```python
from build123d import *

# Parameters (mm, degrees)
SKETCH1_R           = 0.5
BOSS_EXTRUDE1_DEPTH = 2
CUT_EXTRUDE1_DEPTH  = 2
FILLET1_R           = 1
SKETCH4_W           = 2
SKETCH4_H           = 16.2
BOSS_EXTRUDE2_DEPTH = 12


with BuildPart() as part:
    # Sketch1 → Boss-Extrude1 (new body)
    # profile 1 of 3: a face of its own
    with BuildSketch(Plane(origin=(0, -1346.908376945, 0), x_dir=(1, 0, 0), z_dir=(0, 1, 0))):
        Polygon((-1025.832273514, 2000), (-1025.832273514, 1981.9), (-1023.832273514, 1981.9), (-1023.832273514, 2004), (-1027.832273514, 2004), (-1027.832273514, 2002), (-1068.432273514, 2002), (-1068.432273514, 2004), (-1072.432273514, 2004), (-1072.432273514, 1991.5), (-1070.432273514, 1991.5), (-1070.432273514, 2000), align=None)
        with Locations(Location((-1070.432273514, 2002, 0), (0, 0, 270))):
            Circle(SKETCH1_R, mode=Mode.SUBTRACT)
        with Locations(Location((-1025.832273514, 2002, 0), (0, 0, 270))):
            Circle(SKETCH1_R, mode=Mode.SUBTRACT)
    # profile 2 of 3: a face of its own
    with BuildSketch(Plane(origin=(0, -1346.908376945, 0), x_dir=(1, 0, 0), z_dir=(0, 1, 0))):
        Polygon((-1023.832273514, 1981.9), (-1023.832273514, 1967.9), (-1025.832273514, 1967.9), (-1025.832273514, 1966.4), (-1070.432273514, 1966.4), (-1070.432273514, 1974.9), (-1072.432273514, 1974.9), (-1072.432273514, 1991.5), (-1070.432273514, 1991.5), (-1070.432273514, 2000), (-1025.832273514, 2000), (-1025.832273514, 1981.9), align=None)
    # profile 3 of 3: a face of its own
    with BuildSketch(Plane(origin=(0, -1346.908376945, 0), x_dir=(1, 0, 0), z_dir=(0, 1, 0))):
        Polygon((-1027.832273514, 1962.4), (-1023.832273514, 1962.4), (-1023.832273514, 1967.9), (-1025.832273514, 1967.9), (-1025.832273514, 1966.4), (-1070.432273514, 1966.4), (-1070.432273514, 1974.9), (-1072.432273514, 1974.9), (-1072.432273514, 1962.4), (-1068.432273514, 1962.4), (-1068.432273514, 1964.4), (-1027.832273514, 1964.4), align=None)
        with Locations(Location((-1025.832273514, 1964.4, 0), (0, 0, 270))):
            Circle(SKETCH1_R, mode=Mode.SUBTRACT)
        with Locations(Location((-1070.432273514, 1964.4, 0), (0, 0, 270))):
            Circle(SKETCH1_R, mode=Mode.SUBTRACT)
    extrude(amount=BOSS_EXTRUDE1_DEPTH)

    # Sketch3 → Cut-Extrude1 (cut)
    with BuildSketch(Plane(origin=(0, -1344.908376945, 0), x_dir=(1, 0, 0), z_dir=(0, 1, 0))):
        Polygon((-1028.832273514, 1967.9), (-1025.832273514, 1967.9), (-1023.832273514, 1967.9), (-1023.832273514, 1981.9), (-1025.832273514, 1981.9), (-1028.832273514, 1981.9), align=None)
    extrude(amount=-CUT_EXTRUDE1_DEPTH, mode=Mode.SUBTRACT)

    # Fillet1
    fillet1_edges = [part.edges().sort_by_distance(p)[0] for p in [
        (-1028.832273514, -1345.908376945, -1967.9),
        (-1028.832273514, -1345.908376945, -1981.9),
    ]]
    fillet(fillet1_edges, radius=FILLET1_R)

    # Sketch4 → Boss-Extrude2 (add)
    with BuildSketch(Plane.XZ.offset(1346.908376945)):
        with Locations((-1071.432273514, -1983.2)):
            Rectangle(SKETCH4_W, SKETCH4_H)
    extrude(amount=BOSS_EXTRUDE2_DEPTH)


solid = part.part
```
Verification items for the finished model (mm, model axes). A direction names the side the tool comes from. Coordinates: 2 decimals unless noted, no trailing zeros. Order: outer loops, then holes, each group sorted by start corner. A loop starts at its lowest first (then second) coordinate and runs counter-clockwise, first axis right, second up. Notation, with made-up numbers: (20, 19) - (28, 19) arc R30 ccw to (28, 43) - close; hole circle Ø5 at (-25.75, -28.5). An arc over 180 degrees is marked (long way). Return JSON: item names as keys, results as strings.
(1) Go/stop test with flat-tipped pins: pin 1 (2 mm diameter, centred on x = -1062.5, y = -1347, fed in from -Z); pin 2 (21 mm diameter, centred on x = -1059, z = -1993.5, fed in from -Y); pin 3 (4 mm diameter, centred on y = -1350.5, z = -1991.5, fed in from -X); pin 4 (1 mm diameter, centred on x = -1055.5, y = -1346, fed in from +Z). Record where each tip stops, or that it passes through.
Filled sheet:
{"pin 1": "stops at z = -2002", "pin 2": "stops at y = -1346.91", "pin 3": "stops at x = -1072.43", "pin 4": "stops at z = -1964.4"}
(2) Section check A-A, the plane z = -1977. Record the cut outline in (x, y).
Filled sheet:
{"outline": "(-1072.43, -1358.91) - (-1070.43, -1358.91) - (-1070.43, -1346.91) - (-1028.83, -1346.91) - (-1028.83, -1344.91) - (-1072.43, -1344.91) - close"}
(3) Section check D-D, the plane z = -1990. Record the cut outline in (x, y), and give its area (3 significant figures).
Filled sheet:
{"outline": "(-1072.43, -1358.91) - (-1070.43, -1358.91) - (-1070.43, -1346.91) - (-1023.83, -1346.91) - (-1023.83, -1344.91) - (-1072.43, -1344.91) - close", "area": "121 mm^2"}
(4) Section check B-B, the plane y = -1356.75. Record the cut outline in (x, z).
Filled sheet:
{"outline": "(-1072.43, -1991.3) - (-1070.43, -1991.3) - (-1070.43, -1975.1) - (-1072.43, -1975.1) - close"}
(5) Thickness scan on line 1 along Y through (x, z) = (-1052.5, -1995); line 2 along X through (y, z) = (-1353.25, -1977.5); line 3 along Z through (x, y) = (-1044.5, -1345.75). Record the ranges inside material, lowest first.
Filled sheet:
{"line 1": "y = -1346.91 to -1344.91", "line 2": "x = -1072.43 to -1070.43", "line 3": "z = -2002 to -1964.4"}
(6) Mould release check, pull along X, two halves, no side actions. Record for faces 6 (the flat face through (-1070, -1346, -2004)), 7 (the flat face through (-1028.832, -1346, -1975)), 8 (the flat face through (-1027.832, -1346, -2003)): pulls with the +X half, pulls with the -X half, needs draft (parallel to the pull), parting line crosses it, or undercut.
Filled sheet:
{"face 6": "needs draft", "face 7": "pulls with the +X half", "face 8": "undercut"}
(7) Access from +Z, -Z, +X, -X, +Y, -Y to the whole of each face (thin tool, end or side, straight path). Record for faces 1 (the flat face through (-1068.432, -1346, -2003)), 2 (the flat face through (-1071, -1353, -1991.3)), 3 (the flat face through (-1071, -1353, -1975.1)), 4 (the flat face through (-1068.432, -1346, -1963)), 5 (the flat face through (-1026, -1346, -1981.9)).
Filled sheet:
{"face 1": "-Z, +Y, -Y", "face 2": "-Z, +X, -X, -Y", "face 3": "+Z, +X, -X, -Y", "face 4": "+Z, +Y, -Y", "face 5": "+X, +Y, -Y"}
(8) Section check C-C, the plane x = -1042. Record the cut outline in (y, z).
Filled sheet:
{"outline": "(-1346.91, -2002) - (-1344.91, -2002) - (-1344.91, -1964.4) - (-1346.91, -1964.4) - close"}
